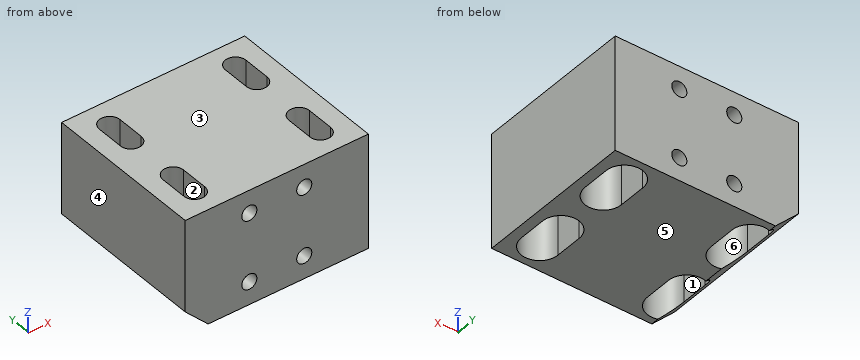
```python
from build123d import *

# Parameters (mm, degrees)
SKETCH1_W                                            = 40
SKETCH1_H                                            = 35
BOSS_EXTRUDE1_DEPTH                                  = 25
CHAMFER1_SIZE                                        = 5
CBORE_FOR_M4_HEXAGON_SOCKET_HEAD_CAP_SCR_D           = 4.5
CBORE_FOR_M4_HEXAGON_SOCKET_HEAD_CAP_SCR_CBORE_D     = 8
CBORE_FOR_M4_HEXAGON_SOCKET_HEAD_CAP_SCR_CBORE_DEPTH = 18
CUT_EXTRUDE1_DEPTH                                   = 33.097507691
CUT_EXTRUDE2_DEPTH                                   = 33.097507691
M4_TAPPED_HOLE1_D                                    = 3.3


with BuildPart() as part:
    # Sketch1 → Boss-Extrude1 (new body)
    with BuildSketch(Plane.XY):
        Rectangle(SKETCH1_W, SKETCH1_H)
    extrude(amount=BOSS_EXTRUDE1_DEPTH)

    # Chamfer1
    chamfer1_edges = [part.edges().sort_by_distance(p)[0] for p in [
        (-20, 0, 0),
    ]]
    chamfer(chamfer1_edges, length=CHAMFER1_SIZE)

    # CBORE for M4 Hexagon socket head cap screws1 (through all)
    with Locations(Plane(origin=(0, 0, 0), x_dir=(-1, 0, 0), z_dir=(0, 0, -1))):
        with Locations((-13.75, 9), (-13.75, -9), (13.75, -9), (13.75, 9)):
            CounterBoreHole(CBORE_FOR_M4_HEXAGON_SOCKET_HEAD_CAP_SCR_D / 2, CBORE_FOR_M4_HEXAGON_SOCKET_HEAD_CAP_SCR_CBORE_D / 2, CBORE_FOR_M4_HEXAGON_SOCKET_HEAD_CAP_SCR_CBORE_DEPTH)

    # Sketch5 → Cut-Extrude1 (cut, through all)
    with BuildSketch(Plane(origin=(0, 0, 18), x_dir=(-1, 0, 0), z_dir=(0, 0, -1))):
        with BuildLine():
            Line((-9.75, 12), (-9.75, 6))
            ThreePointArc((-9.75, 6), (-13.75, 2), (-17.75, 6))
            Line((-17.75, 6), (-17.75, 12))
            ThreePointArc((-17.75, 12), (-13.75, 16), (-9.75, 12))
        make_face()
        with BuildLine():
            Line((-9.75, -12), (-9.75, -6))
            ThreePointArc((-9.75, -6), (-13.75, -2), (-17.75, -6))
            Line((-17.75, -6), (-17.75, -12))
            ThreePointArc((-17.75, -12), (-13.75, -16), (-9.75, -12))
        make_face()
        with BuildLine():
            Line((9.75, 12), (9.75, 6))
            ThreePointArc((9.75, 6), (13.75, 2), (17.75, 6))
            Line((17.75, 6), (17.75, 12))
            ThreePointArc((17.75, 12), (13.75, 16), (9.75, 12))
        make_face()
        with BuildLine():
            Line((9.75, -12), (9.75, -6))
            ThreePointArc((9.75, -6), (13.75, -2), (17.75, -6))
            Line((17.75, -6), (17.75, -12))
            ThreePointArc((17.75, -12), (13.75, -16), (9.75, -12))
        make_face()
    extrude(amount=CUT_EXTRUDE1_DEPTH, mode=Mode.SUBTRACT)

    # Sketch6 → Cut-Extrude2 (cut, through all)
    with BuildSketch(Plane(origin=(0, 0, 18), x_dir=(-1, 0, 0), z_dir=(0, 0, -1))):
        with BuildLine():
            Line((-11.5, 12), (-11.5, 6))
            ThreePointArc((-11.5, 6), (-13.75, 3.75), (-16, 6))
            Line((-16, 6), (-16, 12))
            ThreePointArc((-16, 12), (-13.75, 14.25), (-11.5, 12))
        make_face()
        with BuildLine():
            Line((11.5, 12), (11.5, 6))
            ThreePointArc((11.5, 6), (13.75, 3.75), (16, 6))
            Line((16, 6), (16, 12))
            ThreePointArc((16, 12), (13.75, 14.25), (11.5, 12))
        make_face()
        with BuildLine():
            Line((-11.5, -12), (-11.5, -6))
            ThreePointArc((-11.5, -6), (-13.75, -3.75), (-16, -6))
            Line((-16, -6), (-16, -12))
            ThreePointArc((-16, -12), (-13.75, -14.25), (-11.5, -12))
        make_face()
        with BuildLine():
            Line((11.5, -12), (11.5, -6))
            ThreePointArc((11.5, -6), (13.75, -3.75), (16, -6))
            Line((16, -6), (16, -12))
            ThreePointArc((16, -12), (13.75, -14.25), (11.5, -12))
        make_face()
    extrude(amount=-CUT_EXTRUDE2_DEPTH, mode=Mode.SUBTRACT)

    # M4 Tapped Hole1 (through all)
    with Locations(Plane(origin=(0, 17.5, 0), x_dir=(1, 0, 0), z_dir=(0, 1, 0))):
        with Locations((-6, -5), (-6, -20), (6, -20), (6, -5)):
            Hole(M4_TAPPED_HOLE1_D / 2)


solid = part.part
```
Geometry check sheet. Reference: the model listing, model coordinates, mm. Face numbers are marked on the shaded views. A direction names the side the tool comes from. Coordinates: 2 decimals unless noted, no trailing zeros. Order: outer loops, then holes, each group sorted by start corner. A loop starts at its lowest first (then second) coordinate and runs counter-clockwise, first axis right, second up. Notation, with made-up numbers: M -5.75,72 L 43.25,72 A15 cw 43.25,92 Z; hole C -11.5,17 d6. An arc over 180 degrees is marked long. One line per question, with ' | ' between items. Start each with the question number.
Item 1: Cross-section at A-A on y = 9. Enter the section's corners in (x, z), then the cut area to 3 significant figures.
Item 2: Cross-section at C-C on z = 20. Enter the section's corners in (x, y), then the cut area to 3 significant figures.
Item 3: Gauge pin test, flat ends, axial feed: pin 1 (2.5 mm diameter, centred on x = 14.5, y = 12, fed in from -Z); pin 2 (9 mm diameter, centred on x = -15.5, y = -7, fed in from -Z). Record the tip position at first contact, or that the pin passes through.
Item 4: Material ranges on L1, parallel to Z at x = -6, y = 7; L2, parallel to X at y = -8, z = 5; L3, parallel to X at y = -9, z = 20, recorded low to high. Write a range as [from, to].
Item 5: Cross-section at D-D on y = -0.5. Enter the section's corners in (x, z), then the cut area to 3 significant figures.
Item 6: Draft check along X on the marked faces 4, 5 and 6. Enter one of: pulls with the +X half, pulls with the -X half, needs draft (parallel to the pull), parting line crosses it, or undercut.
Item 7: Set-up check for the marked faces 1, 2 and 3: record each of +Z, -Z, +X, -X, +Y, -Y from which the full face is reachable in a straight line by a thin tool's end or side.
Item 8: Cross-section at B-B on x = 6. Enter the section's corners in (y, z), then the cut area to 3 significant figures.
Findings:
1) outline: M -20,5 L -17.75,2.75 L -17.75,18 L -16,18 L -16,25 L -20,25 Z; M -11.5,18 L -9.75,18 L -9.75,0 L 9.75,0 L 9.75,18 L 11.5,18 L 11.5,25 L -11.5,25 Z; M 16,18 L 17.75,18 L 17.75,0 L 20,0 L 20,25 L 16,25 Z; hole C -6,5 d3.3; hole C -6,20 d3.3; hole C 6,5 d3.3; hole C 6,20 d3.3 | area: 606 mm²
2) outline: M -20,-17.5 L -7.65,-17.5 L -7.65,17.5 L -20,17.5 Z; M -4.35,-17.5 L 4.35,-17.5 L 4.35,17.5 L -4.35,17.5 Z; M 7.65,-17.5 L 20,-17.5 L 20,17.5 L 7.65,17.5 Z; hole M -16,-12 A2.25 ccw -11.5,-12 L -11.5,-6 A2.25 ccw -16,-6 Z; hole M -16,6 A2.25 ccw -11.5,6 L -11.5,12 A2.25 ccw -16,12 Z; hole M 11.5,-12 A2.25 ccw 16,-12 L 16,-6 A2.25 ccw 11.5,-6 Z; hole M 11.5,6 A2.25 ccw 16,6 L 16,12 A2.25 ccw 11.5,12 Z | area: 997 mm²
3) pin 1: passes through | pin 2: stops at z = 0.69
4) L1: z = [0, 3.35], [6.65, 18.35], [21.65, 25] | L2: x = [-20, -17.75], [-9.75, -7.65], [-4.35, 4.35], [7.65, 9.75], [17.75, 20] | L3: x = [-20, -16], [-11.5, -7.65], [-4.35, 4.35], [7.65, 11.5], [16, 20]
5) outline: M -20,5 L -15,0 L 20,0 L 20,25 L -20,25 Z; hole C -6,5 d3.3; hole C -6,20 d3.3; hole C 6,5 d3.3; hole C 6,20 d3.3 | area: 953 mm²
6) face 4: pulls with the -X half | face 5: needs draft | face 6: undercut
7) face 1: -Z | face 2: +Z, -Z | face 3: +Z, +X, -X, +Y, -Y
8) outline: M -17.5,0 L 17.5,0 L 17.5,3.35 L -17.5,3.35 Z; M -17.5,6.65 L 17.5,6.65 L 17.5,18.35 L -17.5,18.35 Z; M -17.5,21.65 L 17.5,21.65 L 17.5,25 L -17.5,25 Z | area: 644 mm²
